Part model, mm, in its own coordinate system. Coordinates: 2 decimals unless noted, no trailing zeros. Loops run counter-clockwise (first coordinate to the right, second up) from the corner with the lowest first, then second, coordinate; pieces in that order, holes last. Notation, with made-up numbers: (36.5, 63.5) - (94.5, 63.5) arc R29 ccw to (94.5, 98.5) - close; hole circle Ø6 at (-3, 30). An arc over 180 degrees is marked (long way). Answer as CSV lines item,"result".
from build123d import *

# Parameters (mm, degrees)
SKETCH1_R               = 5
BOSS_EXTRUDE1_DEPTH     = 141.96
CUT_EXTRUDE1_REACH      = 144.136
SKETCH2_R               = 4
CUT_EXTRUDE2_DEPTH      = 143.135996848
CUT_EXTRUDE2_DEPTH_BACK = 143.135996848
SKETCH5_R               = 1.5


with BuildPart() as part:
    # Sketch1 → Boss-Extrude1 (new body)
    with BuildSketch(Plane.XY):
        with Locations(Location((0, 0, 0), (0, 0, 180))):
            Circle(SKETCH1_R)
    extrude(amount=BOSS_EXTRUDE1_DEPTH)

    # Sketch2 → Cut-Extrude1 (cut, up to next)
    with BuildSketch(Plane.XY.offset(141.96), mode=Mode.PRIVATE) as cut_extrude1_sk1:
        Circle(SKETCH2_R)
    cut_extrude1_tool1 = extrude(cut_extrude1_sk1.sketch, amount=-CUT_EXTRUDE1_REACH, mode=Mode.PRIVATE) & part.part
    add(cut_extrude1_tool1.solids().sort_by_distance((0, 0, 141.96))[0], mode=Mode.SUBTRACT)

    # Sketch5 → Cut-Extrude2 (cut, two sides: drawn at the far end of the back side and taken through both)
    with BuildSketch(Plane(origin=(0, 0, 0), x_dir=(1, 0, 0), z_dir=(0, 1, 0)).offset(-CUT_EXTRUDE2_DEPTH_BACK)):
        with Locations(Location((0, -31.799, 0), (0, 0, 270))):
            Circle(SKETCH5_R)
        with Locations(Location((0, -110.161, 0), (0, 0, 270))):
            Circle(SKETCH5_R)
    extrude(amount=CUT_EXTRUDE2_DEPTH + CUT_EXTRUDE2_DEPTH_BACK, mode=Mode.SUBTRACT)


solid = part.part
Q1. Saw through at B-B (y = 0). Give the cut face in (x, z), then the cut area to 3 significant figures.
Results:
outline,"(-5, 0) - (-4, 0) - (-4, 141.96) - (-5, 141.96) - close; (4, 0) - (5, 0) - (5, 141.96) - (4, 141.96) - close"
area,"284 mm^2"
Q2. Two-plate mould, pull along Y, no slides. Class faces 1 (the face through (-0.867, -3.905, 71.974)), 2 (the face through (5, 0, 70)): released by +Y, released by -Y, zero draft, split by the parting line, or undercut.
Results:
face 1,"undercut"
face 2,"split by the parting line"
Q3. Saw through at C-C (z = 71). Give the cut face in (x, y).
Results:
outline,"circle Ø10 at (0, 0); hole circle Ø8 at (0, 0)"
Q4. Saw through at A-A (x = 0). Give the cut face in (y, z).
Results:
outline,"(-5, 0) - (-4, 0) - (-4, 30.3) - (-5, 30.3) - close; (-5, 33.3) - (-4, 33.3) - (-4, 108.66) - (-5, 108.66) - close; (-5, 111.66) - (-4, 111.66) - (-4, 141.96) - (-5, 141.96) - close; (4, 0) - (5, 0) - (5, 30.3) - (4, 30.3) - close; (4, 33.3) - (5, 33.3) - (5, 108.66) - (4, 108.66) - close; (4, 111.66) - (5, 111.66) - (5, 141.96) - (4, 141.96) - close"
Q5. Flat gauge pins, fed straight in: pin 1 (2 mm diameter, centred on y = -3, z = 54, fed in from +X); pin 2 (3 mm diameter, centred on y = -2.5, z = 19.5, fed in from -X); pin 3 (1.5 mm diameter, centred on y = -3.5, z = 83, fed in from -X). Where does each tip first touch, or does it go through?
Results:
pin 1,"stops at x = 4.58"
pin 2,"stops at x = -4.9"
pin 3,"stops at x = -4.18"
Q6. Wall check: L1, parallel to Z at x = 0, y = -4.6; L2, parallel to X at y = -0.25, z = 13.5; L3, parallel to Y at x = 0, z = 98. Give the ranges that are in metal, low to high.
Results:
L1,"z = 0 to 30.3, 33.3 to 108.66, 111.66 to 141.96"
L2,"x = -4.99 to -3.99, 3.99 to 4.99"
L3,"y = -5 to -4, 4 to 5"
